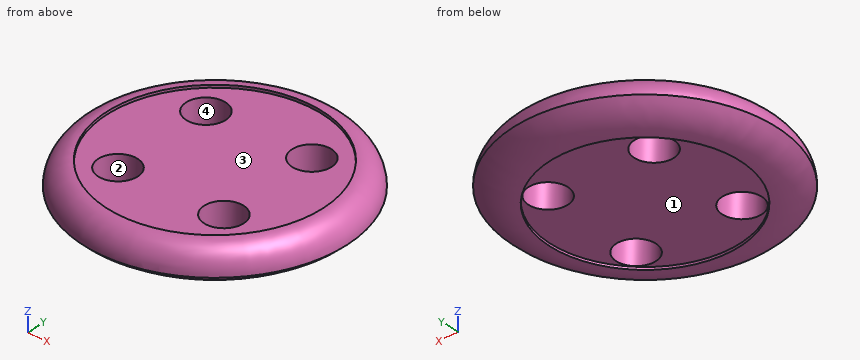
from build123d import *

# Parameters (mm, degrees)
F0_R     = 12.7
F0_R_2   = 1.905
F1_DEPTH = 1.905
F2_R     = 2.286
F4_DEPTH = 0.254
F5_DEPTH = 0.254


# Not quite as in the source:
# - a fillet or chamfer that OpenCascade refuses, or shapes differently, is made with other operations: its cross-section is extruded or revolved along the edge and cut away or added


with BuildPart() as f1:
    # F0 (on Top) → F1 (new body, symmetric)
    with BuildSketch(Plane.XY):
        Circle(F0_R)
        with Locations((-5.08, -5.08)):
            Circle(F0_R_2, mode=Mode.SUBTRACT)
        with Locations((5.08, -5.08)):
            Circle(F0_R_2, mode=Mode.SUBTRACT)
        with Locations((-5.08, 5.08)):
            Circle(F0_R_2, mode=Mode.SUBTRACT)
        with Locations((5.08, 5.08)):
            Circle(F0_R_2, mode=Mode.SUBTRACT)
    extrude(amount=F1_DEPTH, both=True)

    # F2
    f2_edges = [f1.edges().sort_by_distance(p)[0] for p in [
        (-12.7, 0, 1.905),
    ]]
    fillet(f2_edges, radius=F2_R)

    # F3: fillet of radius 4.826 on 1 edges, made by hand

    # F3_s1 → F3_t2 (revolve, cut)
    with BuildSketch(Plane.XZ):
        with BuildLine():
            ThreePointArc((12.7, -0.381), (11.0981307056, -1.5076413266), (9.180472759, -1.905))
            Line((9.180472759, -1.905), (12.7, -1.905))
            Line((12.7, -1.905), (12.7, -0.381))
        make_face()
    revolve(axis=Axis((0, 0, -1.905), (0, 0, 1)), mode=Mode.SUBTRACT)

    # F4 (cut): a face of the model
    f4_faces = [f1.faces().sort_by_distance(p)[0] for p in [
        (0, 0, 1.905),
    ]]
    extrude(f4_faces, amount=-F4_DEPTH, mode=Mode.SUBTRACT)

    # F5 (cut): a face of the model
    f5_faces = [f1.faces().sort_by_distance(p)[0] for p in [
        (0, 0, -1.905),
    ]]
    extrude(f5_faces, amount=-F5_DEPTH, mode=Mode.SUBTRACT)


solid = f1.part
The model under review builds one solid part; all positions refer to its coordinate system, in mm. Face numbers are marked on the shaded views. A direction names the side the tool comes from. Round coordinates to 2 decimals unless told otherwise and drop trailing zeros. Write each loop counter-clockwise with the first axis right and the second up, starting at its lowest first coordinate (ties: lowest second). Pieces come first, ordered by that corner, then holes. Notation, with made-up numbers: M 58,-13.75 L 111,-13.75 A17 cw 111,8.25 Z; hole C 56.5,25 d5. An arc over 180 degrees is marked long. Use a Markdown table: item, result. Add a question column.
Q1. We need section A-A, the plane x = 0. State the section outline as (y, z) points (3 decimals).
Q2. To check wall thickness, follow line 1 (Y direction, x = -3.5, z = 0.95); line 2 (X direction, y = 4.5, z = 0.45); line 3 (X direction, y = -5, z = -0.15). State the ranges of each line that lie inside material, in increasing order.
Q3. We need section D-D, the plane y = -5.08. Count the separate pieces of the cut face and the enclosed holes in it, plus the area to 3 significant figures.
Q4. Insertion check: pin 1 (4 mm diameter, centred on x = 10, y = 6, fed in from -Z); pin 2 (5 mm diameter, centred on x = 3.5, y = 3, fed in from -Z); pin 3 (4.5 mm diameter, centred on x = -5.08, y = 5.08, fed in from +Z). Each pin has a flat end and moves straight along its axis. Give the tip position at first contact, or say it passes through.
Q5. Machinability: for the marked faces 3 and 4, which of the approach directions +Z, -Z, +X, -X, +Y, -Y give a long, thin tool a straight path to every point of the face, cutting with its end or side? Answer none if there is none.
Q6. We need section C-C, the plane z = -0.95. State the section outline as (x, y) points (3 decimals), plus the area to 3 significant figures.
Q7. The part is to be moulded in two halves that separate along Y. For the marked faces 1 and 2, say which applies: pulls with the +Y half, pulls with the -Y half, needs draft (parallel to the pull), parting line crosses it, or undercut.
Findings below:
| question | item | result |
|---|---|---|
| 1 | outline | M -12.7,-0.381 A4.826 ccw -9.18,-1.905 L -9.18,-1.651 L 9.18,-1.651 L 9.18,-1.905 A4.826 ccw 12.7,-0.381 A2.286 ccw 10.414,1.905 L 10.414,1.651 L -10.414,1.651 L -10.414,1.905 A2.286 ccw Z |
| 2 | line 1 | y = -11.76 to -6.14, -4.02 to 4.02, 6.14 to 11.76 |
| 2 | line 2 | x = -11.71 to -6.89, -3.27 to 3.27, 6.89 to 11.71 |
| 2 | line 3 | x = -11.66 to -6.98, -3.18 to 3.18, 6.98 to 11.66 |
| 3 | separate pieces | 3 |
| 3 | enclosed holes | 0 |
| 3 | area | 48.9 mm² |
| 4 | pin 1 | stops at z = -1.88 |
| 4 | pin 2 | stops at z = -1.65 |
| 4 | pin 3 | stops at z = 1.65 |
| 5 | face 3 | +Z |
| 5 | face 4 | +Z, -Z |
| 6 | outline | C 0,0 d24.125; hole C -5.08,-5.08 d3.81; hole C -5.08,5.08 d3.81; hole C 5.08,-5.08 d3.81; hole C 5.08,5.08 d3.81 |
| 6 | area | 412 mm² |
| 7 | face 1 | undercut |
| 7 | face 2 | undercut |
